Part model, mm, in its own coordinate system. Face numbers are marked on the shaded views. Round coordinates to 2 decimals unless told otherwise and drop trailing zeros. Write each loop counter-clockwise with the first axis right and the second up, starting at its lowest first coordinate (ties: lowest second). Pieces come first, ordered by that corner, then holes.
```python
from build123d import *

# Parameters (mm, degrees)
SKETCH1_R           = 1.25
BOSS_EXTRUDE1_DEPTH = 10
BOSS_EXTRUDE2_DEPTH = 20


with BuildPart() as part:
    # Sketch1 → Boss-Extrude1 (new body)
    with BuildSketch(Plane(origin=(0, 0, 0), x_dir=(1, 0, 0), z_dir=(0, 1, 0))):
        with BuildLine():
            Line((0.356274676, 9.337394122), (-12.211586722, -1.118308403))
            ThreePointArc((-12.211586722, -1.118308403), (-12.29724406, -1.631513563), (-12.262730232, -2.150672028))
            Line((-12.262730232, -2.150672028), (6.043725324, -12.823079133))
            Line((6.043725324, -12.823079133), (18.611586722, -2.367376608))
            ThreePointArc((18.611586722, -2.367376608), (18.69724406, -1.854171449), (18.662730232, -1.335012984))
            Line((18.662730232, -1.335012984), (0.356274676, 9.337394122))
        make_face()
        with Locations(Location((-10.05, -1.742842506, 0), (0, 0, 270))):
            Circle(SKETCH1_R, mode=Mode.SUBTRACT)
        with Locations(Location((16.45, -1.742842506, 0), (0, 0, 270))):
            Circle(SKETCH1_R, mode=Mode.SUBTRACT)
    extrude(amount=BOSS_EXTRUDE1_DEPTH)

    # Sketch1_3 → Boss-Extrude2 (add)
    with BuildSketch(Plane(origin=(0, 0, 0), x_dir=(1, 0, 0), z_dir=(0, 1, 0))):
        with BuildLine():
            ThreePointArc((2.925, 0), (-0.917768565, 2.777287501), (-2.349068965, -1.742842506))
            Line((-2.349068965, -1.742842506), (2.349068965, -1.742842506))
            ThreePointArc((2.349068965, -1.742842506), (2.777287501, -0.917768565), (2.925, 0))
        make_face()
        with BuildLine():
            Line((2.349068965, -1.742842506), (-2.349068965, -1.742842506))
            ThreePointArc((-2.349068965, -1.742842506), (0, -2.925), (2.349068965, -1.742842506))
        make_face()
    extrude(amount=-BOSS_EXTRUDE2_DEPTH)


solid = part.part
```
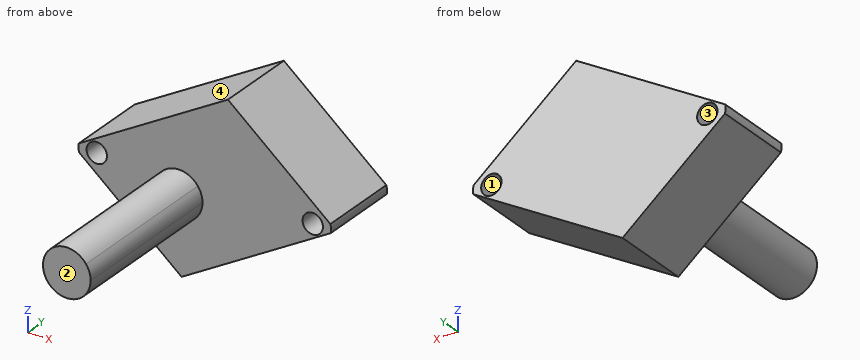
Q1. Wall check: L1, parallel to Y at x = -2, z = -3.25; L2, parallel to Z at x = -11, y = 2.75; L3, parallel to Z at x = 17.5, y = 1.75. Give the ranges that are in metal, low to high.
Values follow:
L1: y = 0 to 10
L2: z = 0.11 to 0.93, 2.56 to 2.89
L3: z = 0.66 to 1.06, 2.42 to 3.29
Q2. Cut at D-D on z = -1.25. Write the cut outline in (x, y), plus the area to 3 significant figures.
Values follow:
outline: (-9.36, 0) - (-2.64, 0) - (-2.64, -20) - (2.64, -20) - (2.64, 0) - (14.23, 0) - (14.23, 10) - (-9.36, 10) - close
area: 342 mm2
Q3. Cut at C-C on y = -7.75. Write the cut outline in (x, z) (3 decimals), plus the area to 3 significant figures.
Values follow:
outline: circle Ø5.85 at (0, 0)
area: 26.9 mm2
Q4. Mould opens along Z. For the marked faces 1, 2, 3 and 4 say: +Z half, -Z half, draft (parallel to the pull), parting line (faces both ways), or undercut.
Values follow:
face 1: undercut
face 2: draft
face 3: undercut
face 4: +Z half
Q5. Drop flat-ended pins along their axis: pin 1 (3 mm diameter, centred on y = 5.5, z = 6.5, fed in from -X); pin 2 (4 mm diameter, centred on x = 16.45, z = 1.74, fed in from -Y); pin 3 (1 mm diameter, centred on x = 10, z = -4.5, fed in from +Y). Give the stop position or say it passes through.
Values follow:
pin 1: stops at x = -7.38
pin 2: stops at y = 0
pin 3: passes through
Q6. Cut at B-B on x = 16.45. Write the cut outline in (y, z).
Values follow:
outline: (0, 0.05) - (10, 0.05) - (10, 0.49) - (0, 0.49) - close; (0, 2.99) - (10, 2.99) - (10, 4.17) - (0, 4.17) - close
Q7. Cut at A-A on y = 2. Write the cut outline in (x, z), plus the area to 3 significant figures.
Values follow:
outline: (-12.26, 2.15) arc R2.25 ccw to (-12.21, 1.12) - (0.36, -9.34) - (18.66, 1.34) arc R2.25 ccw to (18.61, 2.37) - (6.04, 12.82) - close; hole circle Ø2.5 at (-10.05, 1.74); hole circle Ø2.5 at (16.45, 1.74)
area: 348 mm2
